For this review, take the finished solid that the model builds, in its own axes (mm). A direction names the side the tool comes from. Coordinates: 2 decimals unless noted, no trailing zeros. Write each loop counter-clockwise with the first axis right and the second up, starting at its lowest first coordinate (ties: lowest second). Pieces come first, ordered by that corner, then holes.
```python
from build123d import *

# Parameters (mm, degrees)
SZKIC1_W                    = 60
SZKIC1_H                    = 60
DODANIE_WYCI_GNI_CIE1_DEPTH = 200
SKORUPA1_T                  = -3
SZKIC2_W                    = 5
SZKIC2_H                    = 5
SZKIC2_R                    = 1
DODANIE_WYCI_GNI_CIE2_DEPTH = 57
SZKIC4_W                    = 5
SZKIC4_H                    = 5
SZKIC4_R                    = 1
DODANIE_WYCI_GNI_CIE3_DEPTH = 57
SZKIC5_W                    = 5
SZKIC5_H                    = 5
SZKIC5_R                    = 1
DODANIE_WYCI_GNI_CIE4_DEPTH = 57
SZKIC6_W                    = 5
SZKIC6_H                    = 5
SZKIC6_R                    = 1
DODANIE_WYCI_GNI_CIE6_DEPTH = 57
SZKIC9_R                    = 12.875
WYTNIJ_WYCI_GNI_CIE1_DEPTH  = 3
SZKIC10_W                   = 31.55
SZKIC10_H                   = 7.6
DODANIE_WYCI_GNI_CIE7_DEPTH = 26.5
SZKIC13_R                   = 1.5
WYTNIJ_WYCI_GNI_CIE4_DEPTH  = 5
WYTNIJ_WYCI_GNI_CIE7_DEPTH  = 10
SZKIC14_R                   = 1.5
WYTNIJ_WYCI_GNI_CIE8_DEPTH  = 5
WYTNIJ_WYCI_GNI_CIE10_DEPTH = 10


with BuildPart() as part:
    # Szkic1 → Dodanie-wyciągnięcie1 (new body)
    with BuildSketch(Plane(origin=(0, 0, 0), x_dir=(1, 0, 0), z_dir=(0, 1, 0))):
        with Locations((30, 30)):
            Rectangle(SZKIC1_W, SZKIC1_H)
    extrude(amount=DODANIE_WYCI_GNI_CIE1_DEPTH)

    # Skorupa1
    skorupa1_openings = [part.faces().sort_by_distance(p)[0] for p in [
        (30, 100, 0),
    ]]
    offset(amount=SKORUPA1_T, openings=skorupa1_openings, kind=Kind.INTERSECTION)

    # Szkic2 → Dodanie-wyciągnięcie2 (add)
    with BuildSketch(Plane.XY.offset(-57)):
        with Locations((5.5, 194.5)):
            Rectangle(SZKIC2_W, SZKIC2_H)
        with Locations(Location((5.5, 194.5, 0), (0, 0, 180))):
            Circle(SZKIC2_R, mode=Mode.SUBTRACT)
    extrude(amount=DODANIE_WYCI_GNI_CIE2_DEPTH)

    # Szkic4 → Dodanie-wyciągnięcie3 (add)
    with BuildSketch(Plane.XY):
        with Locations((54.5, 194.5)):
            Rectangle(SZKIC4_W, SZKIC4_H)
        with Locations((54.5, 194.5)):
            Circle(SZKIC4_R, mode=Mode.SUBTRACT)
    extrude(amount=-DODANIE_WYCI_GNI_CIE3_DEPTH)

    # Szkic5 → Dodanie-wyciągnięcie4 (add)
    with BuildSketch(Plane.XY.offset(-57)):
        with Locations((5.5, 5.5)):
            Rectangle(SZKIC5_W, SZKIC5_H)
        with Locations(Location((5.5, 5.5, 0), (0, 0, 180))):
            Circle(SZKIC5_R, mode=Mode.SUBTRACT)
    extrude(amount=DODANIE_WYCI_GNI_CIE4_DEPTH)

    # Szkic6 → Dodanie-wyciągnięcie6 (add)
    with BuildSketch(Plane.XY.offset(-57)):
        with Locations((54.5, 5.5)):
            Rectangle(SZKIC6_W, SZKIC6_H)
        with Locations(Location((54.5, 5.5, 0), (0, 0, 180))):
            Circle(SZKIC6_R, mode=Mode.SUBTRACT)
    extrude(amount=DODANIE_WYCI_GNI_CIE6_DEPTH)

    # Szkic9 → Wytnij-wyciągnięcie1 (cut)
    with BuildSketch(Plane(origin=(60, 0, 0), x_dir=(0, 0, -1), z_dir=(1, 0, 0))):
        with Locations((34.18, 159.82)):
            Circle(SZKIC9_R)
    extrude(amount=-WYTNIJ_WYCI_GNI_CIE1_DEPTH, mode=Mode.SUBTRACT)

    # Szkic10 → Dodanie-wyciągnięcie7 (add)
    with BuildSketch(Plane(origin=(3, 0, 0), x_dir=(0, 0, -1), z_dir=(1, 0, 0))):
        with Locations((41.225, 173.56)):
            Rectangle(SZKIC10_W, SZKIC10_H)
        with Locations((41.225, 124.96)):
            Rectangle(SZKIC10_W, SZKIC10_H)
    extrude(amount=DODANIE_WYCI_GNI_CIE7_DEPTH)

    # Szkic13 → Wytnij-wyciągnięcie4 (cut)
    with BuildSketch(Plane(origin=(29.5, 0, 0), x_dir=(0, 0, -1), z_dir=(1, 0, 0))):
        with Locations((39.21, 174.36)):
            Circle(SZKIC13_R)
        with Locations((29.42, 174.36)):
            Circle(SZKIC13_R)
    extrude(amount=-WYTNIJ_WYCI_GNI_CIE4_DEPTH, mode=Mode.SUBTRACT)

    # Szkic15 → Wytnij-wyciągnięcie7 (cut)
    with BuildSketch(Plane(origin=(0, 177.36, 0), x_dir=(1, 0, 0), z_dir=(0, 1, 0))):
        Polygon((13, 25.45), (3, 25.45), (3, 49.45), align=None)
    extrude(amount=-WYTNIJ_WYCI_GNI_CIE7_DEPTH, mode=Mode.SUBTRACT)

    # Szkic14 → Wytnij-wyciągnięcie8 (cut)
    with BuildSketch(Plane(origin=(29.5, 0, 0), x_dir=(0, 0, -1), z_dir=(1, 0, 0))):
        with Locations((39.21, 124.16)):
            Circle(SZKIC14_R)
        with Locations((29.42, 124.16)):
            Circle(SZKIC14_R)
    extrude(amount=-WYTNIJ_WYCI_GNI_CIE8_DEPTH, mode=Mode.SUBTRACT)

    # Szkic17 → Wytnij-wyciągnięcie10 (cut)
    with BuildSketch(Plane(origin=(60, 0, 0), x_dir=(0, 0, -1), z_dir=(1, 0, 0))):
        with BuildLine():
            Line((30.43, 172.445), (30.43, 176.755))
            ThreePointArc((30.43, 176.755), (34.18, 180.505), (37.93, 176.755))
            Line((37.93, 176.755), (37.93, 172.445))
            Line((37.93, 172.445), (37.93, 172.13678225))
            Line((37.93, 172.13678225), (30.43, 172.13678225))
            Line((30.43, 172.13678225), (30.43, 172.445))
        make_face()
    extrude(amount=-WYTNIJ_WYCI_GNI_CIE10_DEPTH, mode=Mode.SUBTRACT)


solid = part.part
```
Q1. Clearance check with a flat-ended pin moving along its axis: pin 1 Ø1.6 at (x, y) = (54.5, 194.5) entering from +Z. State where the tip first meets the part, or that it passes through.
Ans:
pin 1: stops at z = -57
Q2. Add section C-C (x = 21). State the section outline as (y, z) points.
Ans:
outline: (0, -60) - (200, -60) - (200, 0) - (197, 0) - (197, -57) - (177.36, -57) - (177.36, -25.45) - (169.76, -25.45) - (169.76, -57) - (128.76, -57) - (128.76, -25.45) - (121.16, -25.45) - (121.16, -57) - (3, -57) - (3, 0) - (0, 0) - close
Q3. Draft analysis for pull direction Z (two halves, no side actions). For faces 3 (the flat face through (30, 3, -29)), 4 (the flat face through (21, 174, -25.45)), 5 (the flat face through (30, 99, -60)), 6 (the cylindrical face through (58.521, 146.955, -33.667)), state which applies: +Z half, -Z half, draft (parallel to the pull), parting line (faces both ways), or undercut.
Ans:
face 3: draft
face 4: +Z half
face 5: -Z half
face 6: undercut
Q4. Add section D-D (y = 80). State the section outline as (x, z) points.
Ans:
outline: (0, -60) - (60, -60) - (60, 0) - (57, 0) - (57, -57) - (3, -57) - (3, 0) - (0, 0) - close
Q5. Add section B-B (z = -12.5). State the section outline as (x, y) points, then the cut area to 3 significant figures.
Ans:
outline: (0, 0) - (60, 0) - (60, 200) - (0, 200) - close; hole (3, 8) - (8, 8) - (8, 3) - (52, 3) - (52, 8) - (57, 8) - (57, 192) - (52, 192) - (52, 197) - (8, 197) - (8, 192) - (3, 192) - close; hole circle Ø2 at (5.5, 5.5); hole circle Ø2 at (5.5, 194.5); hole circle Ø2 at (54.5, 5.5); hole circle Ø2 at (54.5, 194.5)
area: 1,610 mm2
Q6. Tool access review of faces 1 (the flat face through (5, 192, -29)), 2 (the flat face through (30, 0, -30)): name each direction out of +Z, -Z, +X, -X, +Y, -Y from which nothing blocks a thin tool from reaching the whole face with its end or side.
Ans:
face 1: +Z
face 2: +Z, -Z, +X, -X, -Y
Q7. For probe 1 along Z at (x, y) = (26, 174.36); probe 2 along Y at (x, z) = (27, -29.42); probe 3 along X at (y, z) = (5.5, -31), list the stretches that pass through material, from the lowest coordinate up.
Ans:
probe 1: z = -60 to -40.71, -37.71 to -30.92, -27.92 to -25.45
probe 2: y = 0 to 3, 121.16 to 122.66, 125.66 to 128.76, 169.76 to 172.86, 175.86 to 177.36, 197 to 200
probe 3: x = 0 to 4.5, 6.5 to 8, 52 to 53.5, 55.5 to 60
Q8. Add section A-A (y = 159.82). State the section outline as (x, z) points (3 decimals), then the cut area to 3 significant figures.
Ans:
outline: (0, -60) - (60, -60) - (60, -47.055) - (57, -47.055) - (57, -57) - (3, -57) - (3, 0) - (0, 0) - close; (57, -21.305) - (60, -21.305) - (60, 0) - (57, 0) - close
area: 445 mm2
